from build123d import *

# Parameters (mm, degrees)
F2_R     = 8.255
F3_DEPTH = 25.4
F5_DEPTH = 1.905
F6_R     = 0.254


with BuildPart() as f1:
    # F0 (on Front) → F1 (revolve)
    with BuildSketch(Plane.XZ):
        Polygon((-33.775879, 0), (0, 0), (0, 4.7625), (-30.608637, 4.7625), (-31.75, 5.4483), (-31.75, 12.7), (-37.1348, 12.7), (-37.1348, 10.795), (-38.0492, 10.795), (-38.0492, 7.112), align=None)
    revolve(axis=Axis((0, 0, 2.38125), (0, 0, 1)))

    # F2 (on face) → F3 (cut)
    with BuildSketch(Plane.XY.offset(4.7625)):
        with Locations((-12.7, 0)):
            Circle(F2_R)
        with Locations((12.7, 0)):
            Circle(F2_R)
    extrude(amount=-F3_DEPTH, mode=Mode.SUBTRACT)

    # F4 (on face) → F5 (join, through all)
    with BuildSketch(Plane.XY.offset(12.7)):
        with BuildLine():
            ThreePointArc((1.27, -37.113077), (0, -37.1348), (-1.27, -37.113077))
            Line((-1.27, -37.113077), (-1.27, -38.027999))
            ThreePointArc((-1.27, -38.027999), (0, -38.0492), (1.27, -38.027999))
            Line((1.27, -38.027999), (1.27, -37.113077))
        make_face()
    extrude(amount=-F5_DEPTH)

    # F6
    f6_edges = [f1.edges().sort_by_distance(p)[0] for p in [
        (1.27, -37.113077, 11.7475),
        (1.27, -38.027999, 11.7475),
        (-1.27, -38.027999, 11.7475),
        (-1.27, -37.113077, 11.7475),
    ]]
    fillet(f6_edges, radius=F6_R)


solid = f1.part
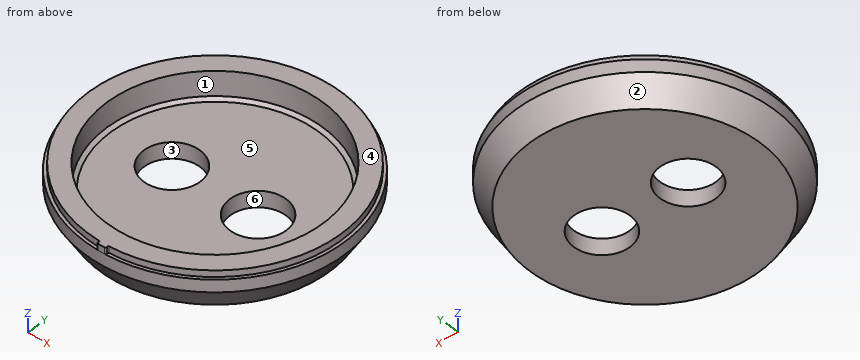
Here's how the part is built. I have some questions about the finished solid (model axes, mm). Face numbers are marked on the shaded views. A direction names the side the tool comes from. Coordinates: 2 decimals unless noted, no trailing zeros. Write each loop counter-clockwise with the first axis right and the second up, starting at its lowest first coordinate (ties: lowest second). Pieces come first, ordered by that corner, then holes.
Item 1: On a 3-axis mill with a long thin cutter (end or side, diameter ignored), from which of +Z, -Z, +X, -X, +Y, -Y can I reach the whole of each face in a straight line? I mean the marked faces 5 and 6. Say none if no direction works.
Item 2: I want a section at C-C on y = -1. Count the separate pieces of the cut face and the enclosed holes in it, and give its area (3 significant figures).
Item 3: Will these pins go through, and if not, where does the flat tip stop? pin 1 (4 mm diameter, centred on y = 24.5, z = 9.5, fed in from -X); pin 2 (4 mm diameter, centred on x = -25, z = 8, fed in from +Y); pin 3 (1 mm diameter, centred on x = 27, z = 1.5, fed in from +Y).
Item 4: If I drill on line 1 (Y direction, x = 0, z = 9.5); line 2 (X direction, y = 7, z = 2); line 3 (Z direction, x = -23, y = 11), over which ranges is the centre line in solid material (lowest first)?
Item 5: I want a section at B-B on z = 8.25. Write out the boundary of the cut face in (x, y), and give its area (3 significant figures).
Item 6: I want a section at D-D on z = 3.5. Write out the boundary of the cut face in (x, y) (3 decimals).
Item 7: If we mould it in two halves opening along X, with no side actions, what happens to the marked faces 1, 2, 3 and 4? For each: +X half, -X half, draft (parallel to the pull), parting line (faces both ways), or undercut.
Findings below:
1. face 5: +Z
1. face 6: +Z, -Z
2. separate pieces: 3
2. enclosed holes: 0
2. area: 273 mm2
3. pin 1: stops at x = -30.68
3. pin 2: stops at y = 30.31
3. pin 3: stops at y = 22.53
4. line 1: y = -38.05 to -31.75, 31.75 to 38.05
4. line 2: x = -34.27 to -17.08, -8.32 to 8.32, 17.08 to 34.27
4. line 3: z = 0 to 4.76
5. outline: circle Ø76.1 at (0, 0); hole circle Ø63.5 at (0, 0)
5. area: 1,380 mm2
6. outline: circle Ø71.758 at (0, 0); hole circle Ø16.51 at (-12.7, 0); hole circle Ø16.51 at (12.7, 0)
7. face 1: undercut
7. face 2: parting line
7. face 3: undercut
7. face 4: draft
